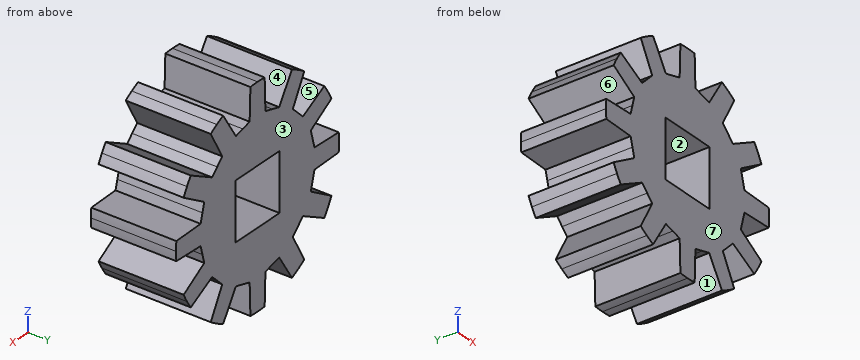
from build123d import *

# Parameters (mm, degrees)
F0_W     = 3.429
F0_H     = 3.429
F1_DEPTH = 5.08


with BuildPart() as f1:
    # F0 (on Front) → F1 (new body)
    with BuildSketch(Plane.XZ):
        with BuildLine():
            ThreePointArc((6.325593, -0.556216), (6.343895, -0.278375), (6.35, 0))
            ThreePointArc((6.35, 0), (6.343895, 0.278375), (6.325593, 0.556216))
            Line((6.325593, 0.556216), (4.437306, 0.613908))
            Line((4.437306, 0.613908), (4.29354, 1.150451))
            Line((4.29354, 1.150451), (4.149774, 1.686993))
            Line((4.149774, 1.686993), (5.756232, 2.6811))
            ThreePointArc((5.756232, 2.6811), (5.633162, 2.930867), (5.499261, 3.175))
            ThreePointArc((5.499261, 3.175), (5.354787, 3.413028), (5.200016, 3.644493))
            Line((5.200016, 3.644493), (3.535866, 2.750313))
            Line((3.535866, 2.750313), (3.14309, 3.14309))
            Line((3.14309, 3.14309), (2.750313, 3.535866))
            Line((2.750313, 3.535866), (3.644493, 5.200016))
            ThreePointArc((3.644493, 5.200016), (3.413028, 5.354787), (3.175, 5.499261))
            ThreePointArc((3.175, 5.499261), (2.930867, 5.633162), (2.6811, 5.756232))
            Line((2.6811, 5.756232), (1.686993, 4.149774))
            Line((1.686993, 4.149774), (1.150451, 4.29354))
            Line((1.150451, 4.29354), (0.613908, 4.437306))
            Line((0.613908, 4.437306), (0.556216, 6.325593))
            ThreePointArc((0.556216, 6.325593), (0.278375, 6.343895), (0, 6.35))
            ThreePointArc((0, 6.35), (-0.278375, 6.343895), (-0.556216, 6.325593))
            Line((-0.556216, 6.325593), (-0.613908, 4.437306))
            Line((-0.613908, 4.437306), (-1.150451, 4.29354))
            Line((-1.150451, 4.29354), (-1.686993, 4.149774))
            Line((-1.686993, 4.149774), (-2.6811, 5.756232))
            ThreePointArc((-2.6811, 5.756232), (-2.930867, 5.633162), (-3.175, 5.499261))
            ThreePointArc((-3.175, 5.499261), (-3.413028, 5.354787), (-3.644493, 5.200016))
            Line((-3.644493, 5.200016), (-2.750313, 3.535866))
            Line((-2.750313, 3.535866), (-3.14309, 3.14309))
            Line((-3.14309, 3.14309), (-3.535866, 2.750313))
            Line((-3.535866, 2.750313), (-5.200016, 3.644493))
            ThreePointArc((-5.200016, 3.644493), (-5.354787, 3.413028), (-5.499261, 3.175))
            ThreePointArc((-5.499261, 3.175), (-5.633162, 2.930867), (-5.756232, 2.6811))
            Line((-5.756232, 2.6811), (-4.149774, 1.686993))
            Line((-4.149774, 1.686993), (-4.29354, 1.150451))
            Line((-4.29354, 1.150451), (-4.437306, 0.613908))
            Line((-4.437306, 0.613908), (-6.325593, 0.556216))
            ThreePointArc((-6.325593, 0.556216), (-6.343895, 0.278375), (-6.35, 0))
            ThreePointArc((-6.35, 0), (-6.343895, -0.278375), (-6.325593, -0.556216))
            Line((-6.325593, -0.556216), (-4.437306, -0.613908))
            Line((-4.437306, -0.613908), (-4.29354, -1.150451))
            Line((-4.29354, -1.150451), (-4.149774, -1.686993))
            Line((-4.149774, -1.686993), (-5.756232, -2.6811))
            ThreePointArc((-5.756232, -2.6811), (-5.633162, -2.930867), (-5.499261, -3.175))
            ThreePointArc((-5.499261, -3.175), (-5.354787, -3.413028), (-5.200016, -3.644493))
            Line((-5.200016, -3.644493), (-3.535866, -2.750313))
            Line((-3.535866, -2.750313), (-3.14309, -3.14309))
            Line((-3.14309, -3.14309), (-2.750313, -3.535866))
            Line((-2.750313, -3.535866), (-3.644493, -5.200016))
            ThreePointArc((-3.644493, -5.200016), (-3.413028, -5.354787), (-3.175, -5.499261))
            ThreePointArc((-3.175, -5.499261), (-2.930867, -5.633162), (-2.6811, -5.756232))
            Line((-2.6811, -5.756232), (-1.686993, -4.149774))
            Line((-1.686993, -4.149774), (-1.150451, -4.29354))
            Line((-1.150451, -4.29354), (-0.613908, -4.437306))
            Line((-0.613908, -4.437306), (-0.556216, -6.325593))
            ThreePointArc((-0.556216, -6.325593), (-0.278375, -6.343895), (0, -6.35))
            ThreePointArc((0, -6.35), (0.278375, -6.343895), (0.556216, -6.325593))
            Line((0.556216, -6.325593), (0.613908, -4.437306))
            Line((0.613908, -4.437306), (1.150451, -4.29354))
            Line((1.150451, -4.29354), (1.686993, -4.149774))
            Line((1.686993, -4.149774), (2.6811, -5.756232))
            ThreePointArc((2.6811, -5.756232), (2.930867, -5.633162), (3.175, -5.499261))
            ThreePointArc((3.175, -5.499261), (3.413028, -5.354787), (3.644493, -5.200016))
            Line((3.644493, -5.200016), (2.750313, -3.535866))
            Line((2.750313, -3.535866), (3.14309, -3.14309))
            Line((3.14309, -3.14309), (3.535866, -2.750313))
            Line((3.535866, -2.750313), (5.200016, -3.644493))
            ThreePointArc((5.200016, -3.644493), (5.354787, -3.413028), (5.499261, -3.175))
            ThreePointArc((5.499261, -3.175), (5.633162, -2.930867), (5.756232, -2.6811))
            Line((5.756232, -2.6811), (4.149774, -1.686993))
            Line((4.149774, -1.686993), (4.29354, -1.150451))
            Line((4.29354, -1.150451), (4.437306, -0.613908))
            Line((4.437306, -0.613908), (6.325593, -0.556216))
        make_face()
        Rectangle(F0_W, F0_H, mode=Mode.SUBTRACT)
    extrude(amount=F1_DEPTH)


solid = f1.part
Work out the finished part from the listing and answer in its coordinate system (mm). Face numbers are marked on the shaded views. A direction names the side the tool comes from. Coordinates: 2 decimals unless noted, no trailing zeros. Loops run counter-clockwise (first coordinate to the right, second up) from the corner with the lowest first, then second, coordinate; pieces in that order, holes last. Notation, with made-up numbers: M 12.5,-17.75 L 65.5,-17.75 A17 cw 65.5,-9.75 Z; hole C -11,72.5 d11. An arc over 180 degrees is marked long. Answer in a Markdown table with one row per item. Add a question column.
1. Consider L1, parallel to Z at x = -3.5, y = -3.5; L2, parallel to X at y = -4.3, z = -0.5. Determine where each line is inside the solid, lowest interval first.
2. Find section C-C, the plane z = 0.25. Write down the section's boundary in (x, y).
3. Find section B-B, the plane z = 4.75. Write down the section's boundary in (x, y).
4. Find section D-D, the plane x = 2.5. Write down the section's boundary in (y, z), then the cut area to 3 significant figures.
5. Flat-ended cylindrical pins translate along their axes: P1, Ø1, axis at y = -4.5, z = 3, coming from the +X side; P2, Ø3, axis at x = 4.5, y = -0.5, coming from the -Z side; P3, Ø1.5, axis at y = -3, z = 5, coming from the +X side. Find the tip coordinate at first contact, or state that the pin passes through.
6. A tool of negligible diameter and unlimited length cuts with its end or side. For the marked faces 1, 2, 3 and 4, from which of +Z, -Z, +X, -X, +Y, -Y can it reach the whole face along a straight path? Write none if from no direction.
7. Find section A-A, the plane x = 5. Write down the section's boundary in (y, z), then the cut area to 3 significant figures.
8. The mould has two halves that part along X. Classify the marked faces 5, 6 and 7: pulls with the +X half, pulls with the -X half, needs draft (parallel to the pull), parting line crosses it, or undercut.
Reported:
| question | item | result |
|---|---|---|
| 1 | L1 | z = -5.3 to -4.93, -2.79 to 2.79, 4.93 to 5.3 |
| 1 | L2 | x = -6.33 to -1.71, 1.71 to 6.33 |
| 2 | outline | M -6.35,-5.08 L -1.71,-5.08 L -1.71,0 L -6.35,0 Z; M 1.71,-5.08 L 6.35,-5.08 L 6.35,0 L 1.71,0 Z |
| 3 | outline | M -3.4,-5.08 L -2.06,-5.08 L -2.06,0 L -3.4,0 Z; M -0.6,-5.08 L 0.6,-5.08 L 0.6,0 L -0.6,0 Z; M 2.06,-5.08 L 3.4,-5.08 L 3.4,0 L 2.06,0 Z |
| 4 | outline | M -5.08,-5.46 L 0,-5.46 L 0,5.46 L -5.08,5.46 Z |
| 4 | area | 55.5 mm^2 |
| 5 | P1 | stops at x = 5.76 |
| 5 | P2 | stops at z = -5.6 |
| 5 | P3 | stops at x = 3.64 |
| 6 | face 1 | -Z, +Y, -Y |
| 6 | face 2 | +Y, -Y |
| 6 | face 3 | +Z, -Z, +X, -X, +Y |
| 6 | face 4 | +Z, +Y, -Y |
| 7 | outline | M -5.08,-3.54 L 0,-3.54 L 0,-2.21 L -5.08,-2.21 Z; M -5.08,-0.6 L 0,-0.6 L 0,0.6 L -5.08,0.6 Z; M -5.08,2.21 L 0,2.21 L 0,3.54 L -5.08,3.54 Z |
| 7 | area | 19.5 mm^2 |
| 8 | face 5 | undercut |
| 8 | face 6 | pulls with the -X half |
| 8 | face 7 | needs draft |
